from build123d import *

# Parameters (mm, degrees)
BOSS_EXTRUDE1_DEPTH = 13
CUT_EXTRUDE1_DEPTH  = 11
SKETCH3_R           = 1.35
CUT_EXTRUDE2_DEPTH  = 75.037152836
SKETCH5_R           = 4.25
SKETCH5_R_2         = 1.35
BOSS_EXTRUDE2_DEPTH = 10
SKETCH6_R           = 3.75
CUT_EXTRUDE3_DEPTH  = 6.6
FILLET1_R           = 1
FILLET2_R           = 4
BOSS_EXTRUDE4_DEPTH = 2.5


with BuildPart() as part:
    # Sketch1 → Boss-Extrude1 (new body)
    with BuildSketch(Plane(origin=(0, 0, 0), x_dir=(1, 0, 0), z_dir=(0, 1, 0))):
        with BuildLine():
            Line((-56.5, 37.5), (56.5, 37.5))
            ThreePointArc((56.5, 37.5), (60.742640687, 35.742640687), (62.5, 31.5))
            Line((62.5, 31.5), (62.5, -31.5))
            ThreePointArc((62.5, -31.5), (60.742640687, -35.742640687), (56.5, -37.5))
            Line((56.5, -37.5), (-56.5, -37.5))
            ThreePointArc((-56.5, -37.5), (-60.742640687, -35.742640687), (-62.5, -31.5))
            Line((-62.5, -31.5), (-62.5, 31.5))
            ThreePointArc((-62.5, 31.5), (-60.742640687, 35.742640687), (-56.5, 37.5))
        make_face()
    extrude(amount=BOSS_EXTRUDE1_DEPTH)

    # Sketch2 → Cut-Extrude1 (cut)
    with BuildSketch(Plane.XZ):
        with BuildLine():
            Line((-60.5, 31.5), (-60.5, -31.5))
            ThreePointArc((-60.5, -31.5), (-59.328427125, -34.328427125), (-56.5, -35.5))
            Line((-56.5, -35.5), (56.5, -35.5))
            ThreePointArc((56.5, -35.5), (59.328427125, -34.328427125), (60.5, -31.5))
            Line((60.5, -31.5), (60.5, 31.5))
            ThreePointArc((60.5, 31.5), (59.328427125, 34.328427125), (56.5, 35.5))
            Line((56.5, 35.5), (-56.5, 35.5))
            ThreePointArc((-56.5, 35.5), (-59.328427125, 34.328427125), (-60.5, 31.5))
        make_face()
    extrude(amount=-CUT_EXTRUDE1_DEPTH, mode=Mode.SUBTRACT)

    # Sketch3 → Cut-Extrude2 (cut, through all)
    with BuildSketch(Plane(origin=(0, 13, 0), x_dir=(1, 0, 0), z_dir=(0, 1, 0))):
        with Locations(Location((-52, -27, 0), (0, 0, 270))):
            Circle(SKETCH3_R)
        with Locations(Location((51, -27, 0), (0, 0, 270))):
            Circle(SKETCH3_R)
        with Locations(Location((51, 26, 0), (0, 0, 270))):
            Circle(SKETCH3_R)
        with Locations(Location((-52, 26, 0), (0, 0, 270))):
            Circle(SKETCH3_R)
    extrude(amount=-CUT_EXTRUDE2_DEPTH, mode=Mode.SUBTRACT)

    # Sketch5 → Boss-Extrude2 (add)
    # profile 1 of 8: a face of its own
    with BuildSketch(Plane.XZ.offset(-11)):
        with BuildLine():
            Line((-52, -30.25), (51, -30.25))
            ThreePointArc((51, -30.25), (49.214642893, -29.856812155), (47.759629651, -28.75))
            Line((47.759629651, -28.75), (-48.759629651, -28.75))
            ThreePointArc((-48.759629651, -28.75), (-50.214642893, -29.856812155), (-52, -30.25))
        make_face()
    # profile 2 of 8: a face of its own
    with BuildSketch(Plane.XZ.offset(-11)):
        with Locations((-52, -26)):
            Circle(SKETCH5_R)
        with Locations(Location((-52, -26, 0), (0, 0, 90))):
            Circle(SKETCH5_R_2, mode=Mode.SUBTRACT)
    # profile 3 of 8: a face of its own
    with BuildSketch(Plane.XZ.offset(-11)):
        with BuildLine():
            ThreePointArc((-54.75, 23.759629651), (-55.856812155, 25.214642893), (-56.25, 27))
            Line((-56.25, 27), (-56.25, -26))
            ThreePointArc((-56.25, -26), (-55.856812155, -24.214642893), (-54.75, -22.759629651))
            Line((-54.75, -22.759629651), (-54.75, 23.759629651))
        make_face()
    # profile 4 of 8: a face of its own
    with BuildSketch(Plane.XZ.offset(-11)):
        with Locations((-52, 27)):
            Circle(SKETCH5_R)
        with Locations(Location((-52, 27, 0), (0, 0, 90))):
            Circle(SKETCH5_R_2, mode=Mode.SUBTRACT)
    # profile 5 of 8: a face of its own
    with BuildSketch(Plane.XZ.offset(-11)):
        with BuildLine():
            ThreePointArc((47.759629651, 29.75), (49.214642893, 30.856812155), (51, 31.25))
            Line((51, 31.25), (-52, 31.25))
            ThreePointArc((-52, 31.25), (-50.214642893, 30.856812155), (-48.759629651, 29.75))
            Line((-48.759629651, 29.75), (47.759629651, 29.75))
        make_face()
    # profile 6 of 8: a face of its own
    with BuildSketch(Plane.XZ.offset(-11)):
        with Locations((51, -26)):
            Circle(SKETCH5_R)
        with Locations(Location((51, -26, 0), (0, 0, 90))):
            Circle(SKETCH5_R_2, mode=Mode.SUBTRACT)
    # profile 7 of 8: a face of its own
    with BuildSketch(Plane.XZ.offset(-11)):
        with BuildLine():
            Line((55.25, -26), (55.25, 27))
            ThreePointArc((55.25, 27), (54.856812155, 25.214642893), (53.75, 23.759629651))
            Line((53.75, 23.759629651), (53.75, -22.759629651))
            ThreePointArc((53.75, -22.759629651), (54.856812155, -24.214642893), (55.25, -26))
        make_face()
    # profile 8 of 8: a face of its own
    with BuildSketch(Plane.XZ.offset(-11)):
        with Locations((51, 27)):
            Circle(SKETCH5_R)
        with Locations(Location((51, 27, 0), (0, 0, 90))):
            Circle(SKETCH5_R_2, mode=Mode.SUBTRACT)
    extrude(amount=BOSS_EXTRUDE2_DEPTH)

    # Sketch6 → Cut-Extrude3 (cut)
    with BuildSketch(Plane(origin=(0, 13, 0), x_dir=(1, 0, 0), z_dir=(0, 1, 0))):
        with Locations(Location((51, 26, 0), (0, 0, 270))):
            Circle(SKETCH6_R)
        with Locations(Location((51, -27, 0), (0, 0, 270))):
            Circle(SKETCH6_R)
        with Locations(Location((-52, 26, 0), (0, 0, 270))):
            Circle(SKETCH6_R)
        with Locations(Location((-52, -27, 0), (0, 0, 270))):
            Circle(SKETCH6_R)
    extrude(amount=-CUT_EXTRUDE3_DEPTH, mode=Mode.SUBTRACT)

    # Fillet1
    fillet1_edges = [part.edges().sort_by_distance(p)[0] for p in [
        (51, 13, 23.25),
        (-52, 13, -29.75),
        (-52, 13, 23.25),
        (51, 13, -29.75),
    ]]
    fillet(fillet1_edges, radius=FILLET1_R)

    # Fillet2
    fillet2_edges = [part.edges().sort_by_distance(p)[0] for p in [
        (60.742640687, 13, 35.742640687),
        (62.5, 13, 0),
        (60.742640687, 13, -35.742640687),
        (0, 13, -37.5),
        (-60.742640687, 13, -35.742640687),
        (-62.5, 13, 0),
        (-60.742640687, 13, 35.742640687),
        (0, 13, 37.5),
    ]]
    fillet(fillet2_edges, radius=FILLET2_R)

    # Sketch8 → Boss-Extrude4 (add)
    with BuildSketch(Plane.XZ.offset(-11)):
        with BuildLine():
            Line((-60.5, 31.5), (-60.5, -31.5))
            ThreePointArc((-60.5, -31.5), (-59.328427125, -34.328427125), (-56.5, -35.5))
            Line((-56.5, -35.5), (56.5, -35.5))
            ThreePointArc((56.5, -35.5), (59.328427125, -34.328427125), (60.5, -31.5))
            Line((60.5, -31.5), (60.5, 31.5))
            ThreePointArc((60.5, 31.5), (59.328427125, 34.328427125), (56.5, 35.5))
            Line((56.5, 35.5), (-56.5, 35.5))
            ThreePointArc((-56.5, 35.5), (-59.328427125, 34.328427125), (-60.5, 31.5))
        make_face()
        with BuildLine():
            Line((55.25, 27), (55.25, -26))
            ThreePointArc((55.25, -26), (54.00520382, -29.00520382), (51, -30.25))
            Line((51, -30.25), (-52, -30.25))
            ThreePointArc((-52, -30.25), (-55.00520382, -29.00520382), (-56.25, -26))
            Line((-56.25, -26), (-56.25, 27))
            ThreePointArc((-56.25, 27), (-55.00520382, 30.00520382), (-52, 31.25))
            Line((-52, 31.25), (51, 31.25))
            ThreePointArc((51, 31.25), (54.00520382, 30.00520382), (55.25, 27))
        make_face(mode=Mode.SUBTRACT)
    extrude(amount=BOSS_EXTRUDE4_DEPTH)


solid = part.part
Could you check a few things on this model? Use its own coordinates, in mm. A direction names the side the tool comes from. Coordinates: 2 decimals unless noted, no trailing zeros. Write each loop counter-clockwise with the first axis right and the second up, starting at its lowest first coordinate (ties: lowest second). Pieces come first, ordered by that corner, then holes. Notation, with made-up numbers: M -38.75,13.5 L 4.25,13.5 A15 ccw 4.25,41.5 Z; hole C -24,25.5 d3. An arc over 180 degrees is marked long. One line per question, with ' | ' between items.
1) Imagine slicing it at B-B, the plane z = -18.5. Write out the boundary of the cut face in (x, y).
Checks:
outline: M -62.5,0 L -60.5,0 L -60.5,8.5 L -56.25,8.5 L -56.25,1 L -54.75,1 L -54.75,11 L 53.75,11 L 53.75,1 L 55.25,1 L 55.25,8.5 L 60.5,8.5 L 60.5,0 L 62.5,0 L 62.5,9 A4 ccw 58.5,13 L -58.5,13 A4 ccw -62.5,9 Z
2) If we mould it in two halves opening along X, with no side actions, what happens to faces 4 (the face through (-1, 4, -37.5)), 5 (the face through (62.5, 4, 0)), 6 (the face through (-59.297, 4.19, 34.359))? For each: released by +X, released by -X, zero draft, split by the parting line, or undercut.
Checks:
face 4: zero draft | face 5: released by +X | face 6: undercut
3) Imagine slicing it at A-A, the plane y = 5. Give the number of separate pieces and of enclosed holes in the cut face, and give its area (3 significant figures).
Checks:
separate pieces: 2 | enclosed holes: 6 | area: 1,410 mm²
4) I need wall thicknesses on probe 1 along X at (y, z) = (3.5, 11); probe 2 along Z at (x, y) = (33, 7); probe 3 along X at (y, z) = (3.55, 27). Which ranges of each line are inside material? Lowest first, please. Write a range as [from, to].
Checks:
probe 1: [-62.5, -60.5], [-56.25, -54.75], [53.75, 55.25], [60.5, 62.5] | probe 2: [-37.5, -35.5], [-30.25, -28.75], [29.75, 31.25], [35.5, 37.5] | probe 3: [-62.5, -60.5], [-56.25, -53.35], [-50.65, -47.75], [46.75, 49.65], [52.35, 55.25], [60.5, 62.5]
5) For pin 1 Ø8.5 at (x, z) = (-52, 27) entering from +Y; pin 2 Ø10 at (x, z) = (-28.5, -30) entering from -Y; pin 3 Ø1.5 at (x, z) = (-22, -12.5) entering from -Y; pin 4 Ø2 at (x, z) = (51, -26) entering from -Y, each with a flat end and sliding along its axis, tell me the tip position at first contact or that it passes through.
Checks:
pin 1: y = 12.87 | pin 2: y = 1 | pin 3: y = 11 | pin 4: through
6) Imagine slicing it at C-C, the plane x = 9. Write out the boundary of the cut face in (y, z), and give its area (3 significant figures).
Checks:
outline: M 0,-37.5 L 9,-37.5 A4 ccw 13,-33.5 L 13,33.5 A4 ccw 9,37.5 L 0,37.5 L 0,35.5 L 8.5,35.5 L 8.5,31.25 L 1,31.25 L 1,29.75 L 11,29.75 L 11,-28.75 L 1,-28.75 L 1,-30.25 L 8.5,-30.25 L 8.5,-35.5 L 0,-35.5 Z | area: 241 mm²
7) For faces 1 (the face through (1, 13, 0)), 2 (the face through (-54, 6.4, -26)), 3 (the face through (-59.359, 4.19, -34.297)), which set-ups out of +Z, -Z, +X, -X, +Y, -Y let a thin tool reach every point of the face, with its end or its side?
Checks:
face 1: +Z, -Z, +X, -X, +Y | face 2: +Y | face 3: -Y
